Verification items for the finished model (mm, model axes). A direction names the side the tool comes from. Coordinates: 2 decimals unless noted, no trailing zeros. Write each loop counter-clockwise with the first axis right and the second up, starting at its lowest first coordinate (ties: lowest second). Pieces come first, ordered by that corner, then holes. Notation, with made-up numbers: (47, 22.5) -> (105, 22.5) arc R11 ccw to (105, 27.5) -> close; hole circle Ø5 at (-21.5, 66). An arc over 180 degrees is marked (long way). Use CSV: the item, a comma, the result in double quotes.
```python
from build123d import *

# Parameters (mm, degrees)
EXTRUDE_3_DEPTH    = 3
FILLET1_R          = 15
SKETCH1_W          = 15
SKETCH1_H          = 40
SKETCH1_W_2        = 3
SKETCH1_H_2        = 20
CUT_EXTRUDE1_DEPTH = 10


with BuildPart() as part:
    # Эскиз4 → Бобышка-Вытянуть3 (new body)
    with BuildSketch(Plane(origin=(0, 0, 0), x_dir=(1, 0, 0), z_dir=(0, 1, 0))):
        Polygon((0, 52), (0, 0), (52, 0), (52, 3), (55, 3), (58, 3), (58, 0), (110, 0), (110, 52), (107, 52), (107, 55), (107, 58), (110, 58), (110, 110), (58, 110), (58, 107), (55, 107), (52, 107), (52, 110), (0, 110), (0, 58), (3, 58), (3, 55), (3, 52), align=None)
    extrude(amount=EXTRUDE_3_DEPTH)

    # Fillet1
    fillet1_edges = [part.edges().sort_by_distance(p)[0] for p in [
        (110, 1.5, 0),
        (0, 1.5, 0),
        (0, 1.5, -110),
        (110, 1.5, -110),
    ]]
    fillet(fillet1_edges, radius=FILLET1_R)

    # Sketch1 → Cut-Extrude1 (cut)
    with BuildSketch(Plane(origin=(0, 3, 0), x_dir=(1, 0, 0), z_dir=(0, 1, 0))):
        with Locations((26.5, 55)):
            Rectangle(SKETCH1_W, SKETCH1_H)
        with Locations((55, 55)):
            Rectangle(SKETCH1_W_2, SKETCH1_H_2)
        with Locations((83.5, 55)):
            Rectangle(SKETCH1_W, SKETCH1_H)
    extrude(amount=-CUT_EXTRUDE1_DEPTH, mode=Mode.SUBTRACT)


solid = part.part
```
1) Scan lines: L1, parallel to X at y = 2.5, z = -71; L2, parallel to X at y = 1.25, z = -59; L3, parallel to Z at x = 23, y = 0.75. Record each from-to range of solid material in increasing order.
Return value:
L1,"0 to 19, 34 to 76, 91 to 110"
L2,"0 to 19, 34 to 53.5, 56.5 to 76, 91 to 110"
L3,"-110 to -75, -35 to 0"
2) Gauge pin test, flat ends, axial feed: pin 1 (1.5 mm diameter, centred on x = 54.5, y = 2, fed in from +Z); pin 2 (1.5 mm diameter, centred on x = 54.5, y = 2, fed in from -Z); pin 3 (1.5 mm diameter, centred on y = 1.5, z = -55.5, fed in from -X). Record the tip position at first contact, or that the pin passes through.
Return value:
pin 1,"z = -3"
pin 2,"z = -107"
pin 3,"x = 3"
3) Cross-section at B-B (z = -54). Record the boundary of the cut face in (x, y), plus the area to 3 significant figures.
Return value:
outline,"(3, 0) -> (19, 0) -> (19, 3) -> (3, 3) -> close; (34, 0) -> (53.5, 0) -> (53.5, 3) -> (34, 3) -> close; (56.5, 0) -> (76, 0) -> (76, 3) -> (56.5, 3) -> close; (91, 0) -> (107, 0) -> (107, 3) -> (91, 3) -> close"
area,"213 mm2"
4) Set-up check for faces 1 (the flat face through (3, 1, -55)), 2 (the flat face through (26, 2, -35)), 3 (the flat face through (55, 1, -3)), 4 (the flat face through (108, 1, -58)): record each of +Z, -Z, +X, -X, +Y, -Y from which the full face is reachable in a straight line by a thin tool's end or side.
Return value:
face 1,"-X, +Y, -Y"
face 2,"+Y, -Y"
face 3,"+Z, +Y, -Y"
face 4,"+X, +Y, -Y"
5) Cross-section at D-D (y = 2.1). Give the number of separate pieces and of enclosed holes in the cut face, plus the area to 3 significant figures.
Return value:
separate pieces,"1"
enclosed holes,"3"
area,"10,600 mm2"
6) Mould release check, pull along X, two halves, no side actions. Record for faces 5 (the flat face through (53.5, 2, -55)), 6 (the flat face through (2, 1, -52)), 7 (the flat face through (110, 1, -76)), 8 (the flat face through (55, 1, -107)): released by +X, released by -X, zero draft, split by the parting line, or undercut.
Return value:
face 5,"undercut"
face 6,"zero draft"
face 7,"released by +X"
face 8,"undercut"
7) Cross-section at A-A (z = -72). Record the boundary of the cut face in (x, y).
Return value:
outline,"(0, 0) -> (19, 0) -> (19, 3) -> (0, 3) -> close; (34, 0) -> (76, 0) -> (76, 3) -> (34, 3) -> close; (91, 0) -> (110, 0) -> (110, 3) -> (91, 3) -> close"
8) Cross-section at C-C (x = 28). Record the boundary of the cut face in (y, z).
Return value:
outline,"(0, -110) -> (3, -110) -> (3, -75) -> (0, -75) -> close; (0, -35) -> (3, -35) -> (3, 0) -> (0, 0) -> close"
